Autodesk Inventor part; units mm, degrees
ref_plane "YZ Plane" through (0, 0, 0) normal (1, 0, 0) x (0, 1, 0)
ref_plane "XZ Plane" through (0, 0, 0) normal (0, 1, 0) x (-1, 0, 0)
ref_plane "XY Plane" through (0, 0, 0) normal (0, 0, 1) x (1, 0, 0)
sketch "SketchCircles" plane through (0, 0, 0) normal (0, 1, 0) x (-1, 0, 0)
  circle A0 centre (0, 0) radius 12.7
  circle A1 centre (0, 0) radius 6.35
  line L0 (32.5969, -6.35) -> (16.267, -6.35)
  line L1 (16.267, 6.35) -> (32.5969, 6.35)
  line L2 (32.5969, 6.35) -> (32.5969, -6.35)
  line L3 (32.5969, -6.35) -> (15.4107, 6.35) construction
  line L4 (15.4107, -6.35) -> (32.5969, 6.35) construction
  arc A2 (16.267, 6.35) -> (16.267, -6.35) centre (0, 0) ccw
  point P0 (24.0038, 0)
  dimension "d0" = 25.4
  dimension "d1" = 12.7
extrude "Extrusion100" add sketch "SketchCircles" along normal blind 6.35 contours A0 | A1 | L0 A2 L1 L2
sketch "SketchLines" plane through (0, 0, 0) normal (0, -1, 0) x (1, 0, 0)
  line L0 (-17.7365, 0) -> (17.5532, 0)
  line L1 (-0.0917, 17.7823) -> (-0.0917, -17.324)
  point P0 (0, 0)
hole "Hole1" at (0, 0, 0) direction (0, 1, 0) diameter 25.4 depth 3.175
sketch "Sketch3" plane through (0, 3.175, 0) normal (0, -1, 0) x (1, 0, 0)
  circle A0 centre (0, 0) radius 6.35
  dimension "d12" = 12.7
extrude "Extrusion2" add sketch "Sketch3" along normal blind 3.175
chamfer "Chamfer1" distance 1.397 angle 45 1 edges at (0, 0, 12.7)
chamfer "Chamfer2" distance 1.397 angle 45 1 edges at (-6.35, 0, 0)
sketch "Sketch4" plane through (0, 6.35, 0) normal (0, 1, 0) x (1, 0, 0)
  circle A0 centre (0, 0) radius 3.9688
  point P0 (0, 0)
  dimension "d21" = 7.9375
hole "Hole2" at (0, 6.35, 0) direction (0, -1, 0) diameter 6.35 depth 12.7
sketch "Sketch5" plane through (0, 0, 0) normal (0, -1, 0) x (1, 0, 0)
  line L0 (-18.8474, 0) -> (20.3869, 0)
  circle A0 centre (0, 0) radius 6.35
  line L1 (-18.8474, 0) -> (-26.1971, 0)
  line L2 (8.1484, 0) -> (8.1484, 20.5164)
  point P0 (0, 0)
  point P1 (6.35, 0)
hole "Hole3" at (-26.1971, 0, 0) direction (0, 1, 0) diameter 6.35 end through all
ref_plane "Work Plane4" through (8.1484, 0, 0) normal (1, 0, 0) x (0, 0, 1)
split "Split2" plane through (8.1484, 0, 0) removes the side toward (1, 0, 0)
properties part number "tiedown-hook-mount-clip"
Build history of the part. All positions in model axes, mm. A direction names the side the tool comes from. Coordinates: 2 decimals unless noted, no trailing zeros. Order: outer loops, then holes, each group sorted by start corner. A loop starts at its lowest first (then second) coordinate and runs counter-clockwise, first axis right, second up. Notation, with made-up numbers: (67, 86) - (82, 86) arc R16 cw to (82, 110) - close; hole circle Ø11 at (27, 39). An arc over 180 degrees is marked (long way). Write each question's results on one line, items separated by ' | '. Start each with the question number.
Item 1: Mould opens along X. For faces 4 (the face through (-7, 3.175, 0)), 5 (the face through (-32.597, 3, 0)), 6 (the face through (-1.38, 2.3, 6.2)), 7 (the face through (-24, 3, 6.35)) say: released by +X, released by -X, zero draft, split by the parting line, or undercut.
Item 2: Band-saw the part on C-C on x = 0. Write the cut outline in (y, z) (3 decimals).
Item 3: Band-saw the part on A-A on z = 0. Write the cut outline in (x, y) (3 decimals), and give its area (3 significant figures).
Item 4: Tool access for faces 1 (the face through (-12.694, 2.298, -0.403)), 2 (the face through (-25, 3, -6.35)), 3 (the face through (-6.29, 3.13, -16.29)): list every direction of +Z, -Z, +X, -X, +Y, -Y with a clear straight run to the whole face (end or side of a thin tool).
Item 5: Band-saw the part on B-B on y = 0.5. Write the cut outline in (x, z) (3 decimals), and give its area (3 significant figures).
Item 6: Band-saw the part on D-D on y = 4.25. Write the cut outline in (x, z) (3 decimals), and give its area (3 significant figures).
Item 7: Flat gauge pins, fed straight in: pin 1 (12 mm diameter, centred on x = -24, z = 13.5, fed in from +Y); pin 2 (8 mm diameter, centred on x = -24.5, z = -7, fed in from -Y); pin 3 (2 mm diameter, centred on x = -10, z = 7.5, fed in from -Y); pin 4 (1 mm diameter, centred on y = 1, z = 2, fed in from +X). Where does each tip first touch, or does it go through?
Item 8: Wall check: probe 1 along X at (y, z) = (5, 0) (3 decimals); probe 2 along Z at (x, y) = (4, 2); probe 3 along Z at (x, y) = (-17.5, 0.5). Give the ranges that are in metal, low to high. Write a range as [from, to].
Numbers:
1) face 4: undercut | face 5: released by -X | face 6: undercut | face 7: zero draft
2) outline: (0, -17.462) - (6.35, -17.462) - (6.35, -3.175) - (0, -3.175) - (0, -4.953) - (1.397, -6.35) - (3.175, -6.35) - (3.175, -12.7) - (1.397, -12.7) - (0, -14.097) - close; (0, 3.175) - (6.35, 3.175) - (6.35, 17.462) - (0, 17.462) - (0, 14.097) - (1.397, 12.7) - (3.175, 12.7) - (3.175, 6.35) - (1.397, 6.35) - (0, 4.953) - close
3) outline: (-32.597, 0) - (-29.372, 0) - (-29.372, 6.35) - (-32.597, 6.35) - close; (-23.022, 0) - (-14.097, 0) - (-12.7, 1.397) - (-12.7, 3.175) - (-6.35, 3.175) - (-6.35, 1.397) - (-4.953, 0) - (-3.175, 0) - (-3.175, 6.35) - (-23.022, 6.35) - close; (3.175, 0) - (4.953, 0) - (6.35, 1.397) - (6.35, 3.175) - (8.148, 3.175) - (8.148, 6.35) - (3.175, 6.35) - close | area: 149 mm^2
4) face 1: -Y | face 2: -Z, -X, +Y, -Y | face 3: -Z, +Y, -Y
5) outline: (-32.597, -6.35) - (-16.267, -6.35) arc R17.462 ccw to (8.148, -15.445) - (8.148, -10.885) arc R13.597 cw (long way) to (8.148, 10.885) - (8.148, 15.445) arc R17.462 ccw to (-16.267, 6.35) - (-32.597, 6.35) - close; circle Ø10.906 at (0, 0); hole circle Ø6.35 at (-26.197, 0); hole circle Ø6.35 at (0, 0) | area: 482 mm^2
6) outline: (-32.597, -6.35) - (-16.267, -6.35) arc R17.462 ccw to (8.148, -15.445) - (8.148, 15.445) arc R17.462 ccw to (-16.267, 6.35) - (-32.597, 6.35) - close; hole circle Ø6.35 at (-26.197, 0); hole circle Ø6.35 at (0, 0) | area: 887 mm^2
7) pin 1: through | pin 2: y = 0 | pin 3: y = 0.6 | pin 4: x = 6.12
8) probe 1: [-32.597, -29.372], [-23.022, -3.175], [3.175, 8.148] | probe 2: [-17, -12.05], [-4.93, 4.93], [12.05, 17] | probe 3: [-6.35, 6.35]
